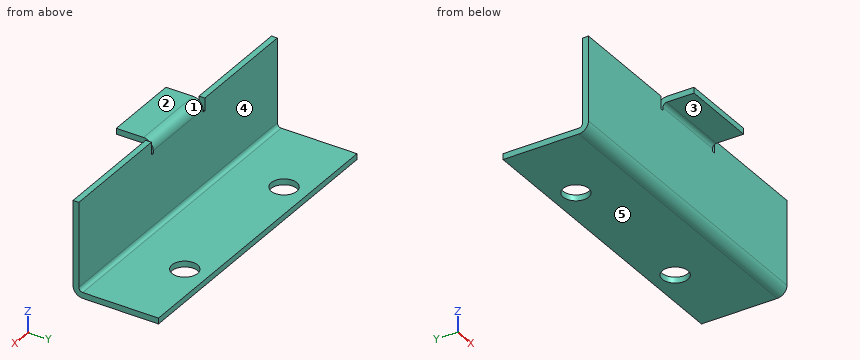
from build123d import *

# Parameters (mm, degrees)
SM_BASE_FLANGE_1_DEPTH            = 40
SM_EDGE_FLANGE_1_STRIP_W          = 8
SM_EDGE_FLANGE_1_STRIP_H          = 1.5
SM_EDGE_FLANGE_1_STRIP_CUT_DEPTH  = 20
SM_EDGE_FLANGE_1_RELIEF_W         = 8.75
SM_EDGE_FLANGE_1_RELIEF_H         = 0.75
SM_EDGE_FLANGE_1_RELIEF_CUT_DEPTH = 1.5
SM_EDGE_FLANGE_1_DEPTH            = 20
HOLE_WIZARD_M6_1_D                = 6.6


# Sheet-metal steps are written as plain solids
with BuildPart() as part:
    # Sketch 1 → 基体-法兰1 (new, symmetric)
    with BuildSketch(Plane(origin=(0, 0, 0), x_dir=(0, 0, -1), z_dir=(1, 0, 0))):
        with BuildLine():
            Line((0, 0), (0, -19.5))
            ThreePointArc((0, -19.5), (-0.732233047, -21.267766953), (-2.5, -22))
            Line((-2.5, -22), (-24.2, -22))
            Line((-24.2, -22), (-24.2, -20.5))
            Line((-24.2, -20.5), (-2.5, -20.5))
            ThreePointArc((-2.5, -20.5), (-1.792893219, -20.207106781), (-1.5, -19.5))
            Line((-1.5, -19.5), (-1.5, 0))
            Line((-1.5, 0), (0, 0))
        make_face()
    extrude(amount=SM_BASE_FLANGE_1_DEPTH, both=True)

    # 边线-法兰1 strip (across the edge) → 边线-法兰1 strip cut (cut)
    with BuildSketch(Plane(origin=(10, -22, 24.2), x_dir=(0, 0, -1), z_dir=(-1, 0, 0))):
        with Locations((-1.5, -0.75)):
            Rectangle(SM_EDGE_FLANGE_1_STRIP_W, SM_EDGE_FLANGE_1_STRIP_H)
    extrude(amount=SM_EDGE_FLANGE_1_STRIP_CUT_DEPTH, mode=Mode.SUBTRACT)

    # 边线-法兰1 relief (on the sheet) → 边线-法兰1 relief cut (cut)
    with BuildSketch(Plane(origin=(10, -22, 21.7), x_dir=(0, 0, -1), z_dir=(0, -1, 0))):
        with Locations((-3.625, 0.375)):
            Rectangle(SM_EDGE_FLANGE_1_RELIEF_W, SM_EDGE_FLANGE_1_RELIEF_H)
        with Locations((-3.625, -20.375)):
            Rectangle(SM_EDGE_FLANGE_1_RELIEF_W, SM_EDGE_FLANGE_1_RELIEF_H)
    extrude(amount=-SM_EDGE_FLANGE_1_RELIEF_CUT_DEPTH, mode=Mode.SUBTRACT)

    # 边线-法兰1 section (across the edge) → 边线-法兰1 (add)
    with BuildSketch(Plane(origin=(10, -22, 24.2), x_dir=(0, 0, -1), z_dir=(-1, 0, 0))):
        with BuildLine():
            Line((0, 1), (0, 8))
            Line((0, 8), (1.5, 8))
            Line((1.5, 8), (1.5, 1))
            ThreePointArc((1.5, 1), (1.792893219, 0.292893219), (2.5, 0))
            Line((2.5, 0), (2.5, -1.5))
            ThreePointArc((2.5, -1.5), (0.732233047, -0.767766953), (0, 1))
        make_face()
    extrude(amount=SM_EDGE_FLANGE_1_DEPTH)

    # M6 间隙孔1 (through all)
    with Locations(Plane(origin=(0, 0, 0), x_dir=(-1, 0, 0), z_dir=(0, 0, -1))):
        with Locations((-20, -6), (20, -6)):
            Hole(HOLE_WIZARD_M6_1_D / 2)


solid = part.part
Input: part model. Units: mm. Frame: model coordinates. Face numbers are marked on the shaded views. A direction names the side the tool comes from. Give positions to 0.01 mm unless a question says otherwise; leave off trailing zeros. Write each loop counter-clockwise with the first axis right and the second up, starting at its lowest first coordinate (ties: lowest second). Pieces come first, ordered by that corner, then holes.
Q1. Set-up query: the marked faces 3, 4 and 5. Return all of +Z, -Z, +X, -X, +Y, -Y with unobstructed straight access to the full face (end or side cutting, diameter ignored); none if empty.
Q2. Section C-C, the plane x = 0.5. Output: boundary loops of the cut face in (y, z), plus the area to 3 significant figures.
Q3. Section A-A, the plane y = -6. Output: boundary loops of the cut face in (x, z), plus the area to 3 significant figures.
Q4. Section D-D, the plane z = 4.25. Output: boundary loops of the cut face in (x, y).
Q5. Section B-B, the plane x = 20. Output: boundary loops of the cut face in (y, z), plus the area to 3 significant figures.
Q6. Material intervals for probe 1 along Y at (x, z) = (14, 5); probe 2 along Y at (x, z) = (-20, 0.4); probe 3 along Y at (x, z) = (-20, 0.7), sorted ascending.
Q7. First-contact query: P1, Ø1, axis at y = -23.5, z = 23, coming from the -X side; P2, Ø11, axis at x = -3.5, z = 10, coming from the +Y side; P3, Ø4, axis at x = -26, y = -14.5, coming from the +Z side; P4, Ø4, axis at x = 20, y = -6, coming from the -Z side. Flat tips, straight axial feed; report the tip coordinate or a pass-through.
Q8. Pull-direction query (X, two-part tool) for the marked faces 1 and 2; classes: pulls with the +X half, pulls with the -X half, needs draft (parallel to the pull), parting line crosses it, or undercut.
Filled in:
1. face 3: -Z, +X, -X, -Y
1. face 4: +Z, +X, -X, +Y
1. face 5: -Z, +X, -X, +Y, -Y
2. outline: (-30, 22.7) - (-23, 22.7) arc R1 cw to (-22, 21.7) - (-22, 2.5) arc R2.5 ccw to (-19.5, 0) - (0, 0) - (0, 1.5) - (-19.5, 1.5) arc R1 cw to (-20.5, 2.5) - (-20.5, 21.7) arc R2.5 ccw to (-23, 24.2) - (-30, 24.2) - close
2. area: 76.8 mm2
3. outline: (-40, 0) - (-23.3, 0) - (-23.3, 1.5) - (-40, 1.5) - close; (-16.7, 0) - (16.7, 0) - (16.7, 1.5) - (-16.7, 1.5) - close; (23.3, 0) - (40, 0) - (40, 1.5) - (23.3, 1.5) - close
3. area: 100 mm2
4. outline: (-40, -22) - (40, -22) - (40, -20.5) - (-40, -20.5) - close
5. outline: (-22, 2.5) arc R2.5 ccw to (-19.5, 0) - (-9.3, 0) - (-9.3, 1.5) - (-19.5, 1.5) arc R1 cw to (-20.5, 2.5) - (-20.5, 24.2) - (-22, 24.2) - close; (-2.7, 0) - (0, 0) - (0, 1.5) - (-2.7, 1.5) - close
5. area: 56.0 mm2
6. probe 1: y = -22 to -20.5
6. probe 2: y = -20.86 to -9.3, -2.7 to 0
6. probe 3: y = -21.23 to -9.3, -2.7 to 0
7. P1: stops at x = -10
7. P2: stops at y = -20.5
7. P3: stops at z = 1.5
7. P4: passes through
8. face 1: undercut
8. face 2: needs draft
